```python
from build123d import *

# Parameters (mm, degrees)
BOSS_EXTRUDE1_DEPTH = 3
SKETCH2_W           = 3
SKETCH2_H           = 36.5
SKETCH2_W_2         = 30
SKETCH2_H_2         = 3
CUT_EXTRUDE1_DEPTH  = 3


with BuildPart() as part:
    # Sketch1 → Boss-Extrude1 (new body)
    with BuildSketch(Plane.XY):
        with BuildLine():
            Line((-26.5, 101.5), (26.5, 101.5))
            ThreePointArc((26.5, 101.5), (30.742640687, 99.742640687), (32.5, 95.5))
            Line((32.5, 95.5), (32.5, -95.5))
            ThreePointArc((32.5, -95.5), (30.742640687, -99.742640687), (26.5, -101.5))
            Line((26.5, -101.5), (-26.5, -101.5))
            ThreePointArc((-26.5, -101.5), (-30.742640687, -99.742640687), (-32.5, -95.5))
            Line((-32.5, -95.5), (-32.5, 95.5))
            ThreePointArc((-32.5, 95.5), (-30.742640687, 99.742640687), (-26.5, 101.5))
        make_face()
    extrude(amount=BOSS_EXTRUDE1_DEPTH)

    # Sketch2 → Cut-Extrude1 (cut)
    with BuildSketch(Plane.XY.offset(3)):
        with Locations((26, -38.25)):
            Rectangle(SKETCH2_W, SKETCH2_H)
        with Locations((0, 95)):
            Rectangle(SKETCH2_W_2, SKETCH2_H_2)
        with Locations((26, 38.25)):
            Rectangle(SKETCH2_W, SKETCH2_H)
        with Locations((0, -95)):
            Rectangle(SKETCH2_W_2, SKETCH2_H_2)
        with Locations((-26, 38.25)):
            Rectangle(SKETCH2_W, SKETCH2_H)
        with Locations((-26, -38.25)):
            Rectangle(SKETCH2_W, SKETCH2_H)
    extrude(amount=-CUT_EXTRUDE1_DEPTH, mode=Mode.SUBTRACT)


solid = part.part
```
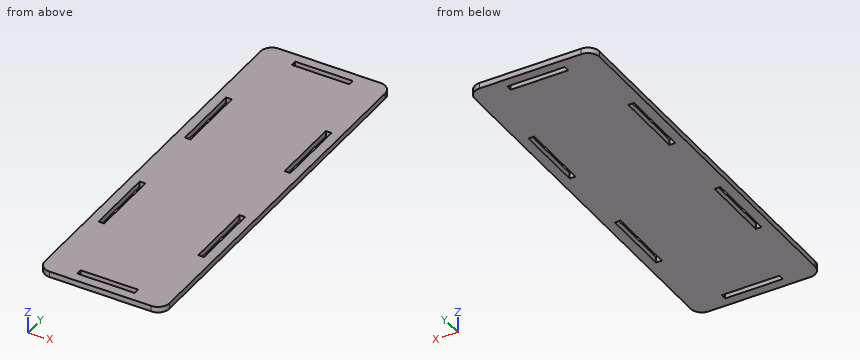
Can you work these out from the model? Positions are in its coordinate system, mm. Give positions to 0.01 mm unless a question says otherwise; leave off trailing zeros. Loops run counter-clockwise (first coordinate to the right, second up) from the corner with the lowest first, then second, coordinate; pieces in that order, holes last. Notation, with made-up numbers: M 0.25,74.25 L 22.25,74.25 A15 cw 22.25,82.25 Z; hole C 67.25,35 d7. An arc over 180 degrees is marked long. One line per item, written item: value.
(1) Suppose I cut it at A-A on x = 0. List the corners of the cut face in (y, z) for me.
Returned:
outline: M -101.5,0 L -96.5,0 L -96.5,3 L -101.5,3 Z; M -93.5,0 L 93.5,0 L 93.5,3 L -93.5,3 Z; M 96.5,0 L 101.5,0 L 101.5,3 L 96.5,3 Z
(2) Suppose I cut it at B-B on z = 2. Count the separate pieces of the cut face and the enclosed holes in it, plus the area to 3 significant figures.
Returned:
separate pieces: 1
enclosed holes: 6
area: 12,500 mm^2
(3) Suppose I cut it at C-C on y = 43. List the corners of the cut face in (x, z) for me, plus the area to 3 significant figures.
Returned:
outline: M -32.5,0 L -27.5,0 L -27.5,3 L -32.5,3 Z; M -24.5,0 L 24.5,0 L 24.5,3 L -24.5,3 Z; M 27.5,0 L 32.5,0 L 32.5,3 L 27.5,3 Z
area: 177 mm^2
(4) I need wall thicknesses on line 1 (X direction, y = -53.5, z = 0.75); line 2 (Y direction, x = 2, z = 1.55); line 3 (Y direction, x = -27, z = 2.05). Which ranges of each line are inside material? Lowest first, please.
Returned:
line 1: -32.5 to -27.5, -24.5 to 24.5, 27.5 to 32.5
line 2: -101.5 to -96.5, -93.5 to 93.5, 96.5 to 101.5
line 3: -101.48 to -56.5, -20 to 20, 56.5 to 101.48
